from build123d import *

# Parameters (mm, degrees)
SKETCH1_W           = 38.1
SKETCH1_H           = 609.6
BOSS_EXTRUDE1_DEPTH = 3.175
FILLET1_R           = 2.54
SKETCH4_R           = 3.175
SKETCH4_R_2         = 6.35
CUT_EXTRUDE1_DEPTH  = 4.175


with BuildPart() as part:
    # Sketch1 → Boss-Extrude1 (new body)
    with BuildSketch(Plane(origin=(0, 0, 0), x_dir=(1, 0, 0), z_dir=(0, 1, 0))):
        with Locations((19.05, 304.8)):
            Rectangle(SKETCH1_W, SKETCH1_H)
    extrude(amount=BOSS_EXTRUDE1_DEPTH)

    # Fillet1
    fillet1_edges = [part.edges().sort_by_distance(p)[0] for p in [
        (38.1, 1.5875, -609.6),
        (38.1, 1.5875, 0),
    ]]
    fillet(fillet1_edges, radius=FILLET1_R)

    # Sketch4 → Cut-Extrude1 (cut, through all)
    with BuildSketch(Plane(origin=(0, 3.175, 0), x_dir=(-1, 0, 0), z_dir=(0, 1, 0))):
        with Locations((-25.4, -152.4)):
            Circle(SKETCH4_R)
        with Locations((-25.4, -203.2)):
            Circle(SKETCH4_R)
        with Locations((-25.4, -254)):
            Circle(SKETCH4_R)
        with Locations((-25.4, -304.8)):
            Circle(SKETCH4_R)
        with Locations((-25.4, -355.6)):
            Circle(SKETCH4_R)
        with Locations((-25.4, -50.8)):
            Circle(SKETCH4_R_2)
        with Locations((-25.4, -101.6)):
            Circle(SKETCH4_R_2)
        with Locations((-25.4, -558.8)):
            Circle(SKETCH4_R_2)
        with Locations((-25.4, -508)):
            Circle(SKETCH4_R_2)
    extrude(amount=-CUT_EXTRUDE1_DEPTH, mode=Mode.SUBTRACT)


solid = part.part
Model file for the job. Use its own axes, mm. Round coordinates to 2 decimals unless told otherwise and drop trailing zeros. Loops run counter-clockwise (first coordinate to the right, second up) from the corner with the lowest first, then second, coordinate; pieces in that order, holes last. Notation, with made-up numbers: (-23.5, 49.5) - (1.5, 49.5) arc R16 cw to (1.5, 80.5) - close; hole circle Ø5 at (5, 24). An arc over 180 degrees is marked (long way). Write each question's results on one line, items separated by ' | '.
(1) Saw through at A-A, the plane z = -508. List the corners of the cut face in (x, y) (3 decimals), then the cut area to 3 significant figures.
Answer below:
outline: (0, 0) - (19.05, 0) - (19.05, 3.175) - (0, 3.175) - close; (31.75, 0) - (38.1, 0) - (38.1, 3.175) - (31.75, 3.175) - close | area: 80.6 mm^2
(2) Mould opens along Z. For faces 1 (the cylindrical face through (21.986, 1.61, -96.246)), 2 (the flat face through (19, 3.175, -309)) say: released by +Z, released by -Z, zero draft, split by the parting line, or undercut.
Answer below:
face 1: undercut | face 2: zero draft
(3) Wall check: L1, parallel to Z at x = 21.5, y = 1.7; L2, parallel to Z at x = 29, y = 0.95; L3, parallel to X at y = 2.45, z = -355.6 (3 decimals). Give the ranges that are in metal, low to high.
Answer below:
L1: z = -609.6 to -563.81, -553.79 to -513.01, -502.99 to -106.61, -96.59 to -55.81, -45.79 to 0 | L2: z = -609.6 to -564.03, -553.57 to -513.23, -502.77 to -106.83, -96.37 to -56.03, -45.57 to 0 | L3: x = 0 to 22.225, 28.575 to 38.1
(4) Saw through at B-B, the plane y = 1.8. Count the separate pieces of the cut face and the enclosed holes in it, then the cut area to 3 significant figures.
Answer below:
separate pieces: 1 | enclosed holes: 9 | area: 22,600 mm^2
